Verification items for the finished model (mm, model axes). Face numbers are marked on the shaded views. Coordinates: 2 decimals unless noted, no trailing zeros. Order: outer loops, then holes, each group sorted by start corner. A loop starts at its lowest first (then second) coordinate and runs counter-clockwise, first axis right, second up. Notation, with made-up numbers: M -30,11.5 L -26,11.5 A25 cw -26,46.5 Z; hole C 11,22.25 d9. An arc over 180 degrees is marked long. Write item = value, one per line.
```python
from build123d import *

# Parameters (mm, degrees)
SKETCH1_R           = 28.5
BOSS_EXTRUDE1_DEPTH = 86
SKETCH2_R           = 27
CUT_EXTRUDE1_DEPTH  = 84
FILLET1_R           = 1
FILLET2_R           = 0.75


with BuildPart() as part:
    # Sketch1 → Boss-Extrude1 (new body)
    with BuildSketch(Plane.XY):
        Circle(SKETCH1_R)
    extrude(amount=BOSS_EXTRUDE1_DEPTH)

    # Sketch2 → Cut-Extrude1 (cut)
    with BuildSketch(Plane.XY.offset(86)):
        Circle(SKETCH2_R)
    extrude(amount=-CUT_EXTRUDE1_DEPTH, mode=Mode.SUBTRACT)

    # Fillet1
    fillet1_edges = [part.edges().sort_by_distance(p)[0] for p in [
        (-28.5, 0, 0),
    ]]
    fillet(fillet1_edges, radius=FILLET1_R)

    # Fillet2
    fillet2_edges = [part.edges().sort_by_distance(p)[0] for p in [
        (-28.5, 0, 86),
        (-27, 0, 86),
    ]]
    fillet(fillet2_edges, radius=FILLET2_R - 0.0001)  # a hair under: the kernel refuses the full size


solid = part.part
```
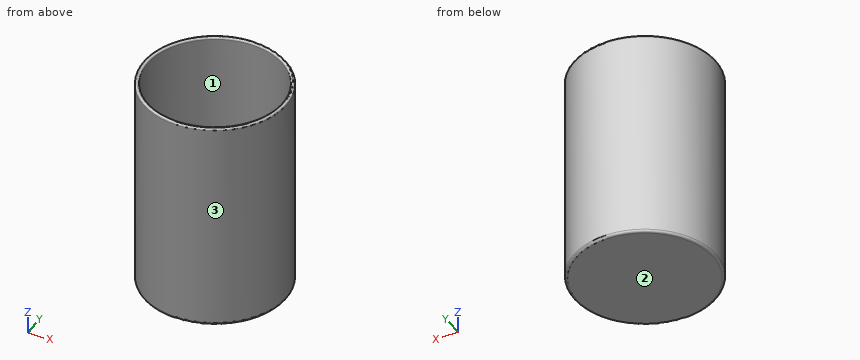
Item 1: Scan lines: L1, parallel to Y at x = 0, z = 45.5; L2, parallel to Z at x = 18, y = 7; L3, parallel to X at y = 1.5, z = 49. Record each from-to range of solid material in increasing order. Write a range as from..to.
Report:
L1 = -28.5..-27, 27..28.5
L2 = 0..2
L3 = -28.46..-26.96, 26.96..28.46
Item 2: Release check for a two-part mould opening along X. For the marked faces 1, 2 and 3 record: pulls with the +X half, pulls with the -X half, needs draft (parallel to the pull), parting line crosses it, or undercut.
Report:
face_1 = undercut
face_2 = needs draft
face_3 = parting line crosses it
Item 3: Sectioned sample at B-B, the plane z = 7. Enter the section's corners in (x, y).
Report:
outline = C 0,0 d57; hole C 0,0 d54
Item 4: Gauge pin test, flat ends, axial feed: pin 1 (5 mm diameter, centred on y = 11.5, z = 55, fed in from -X); pin 2 (1 mm diameter, centred on y = -11.5, z = 67.5, fed in from -X); pin 3 (6 mm diameter, centred on x = 5, z = 76.5, fed in from -Y). Record the tip position at first contact, or that the pin passes through.
Report:
pin_1 = -27.04
pin_2 = -26.29
pin_3 = -28.43
